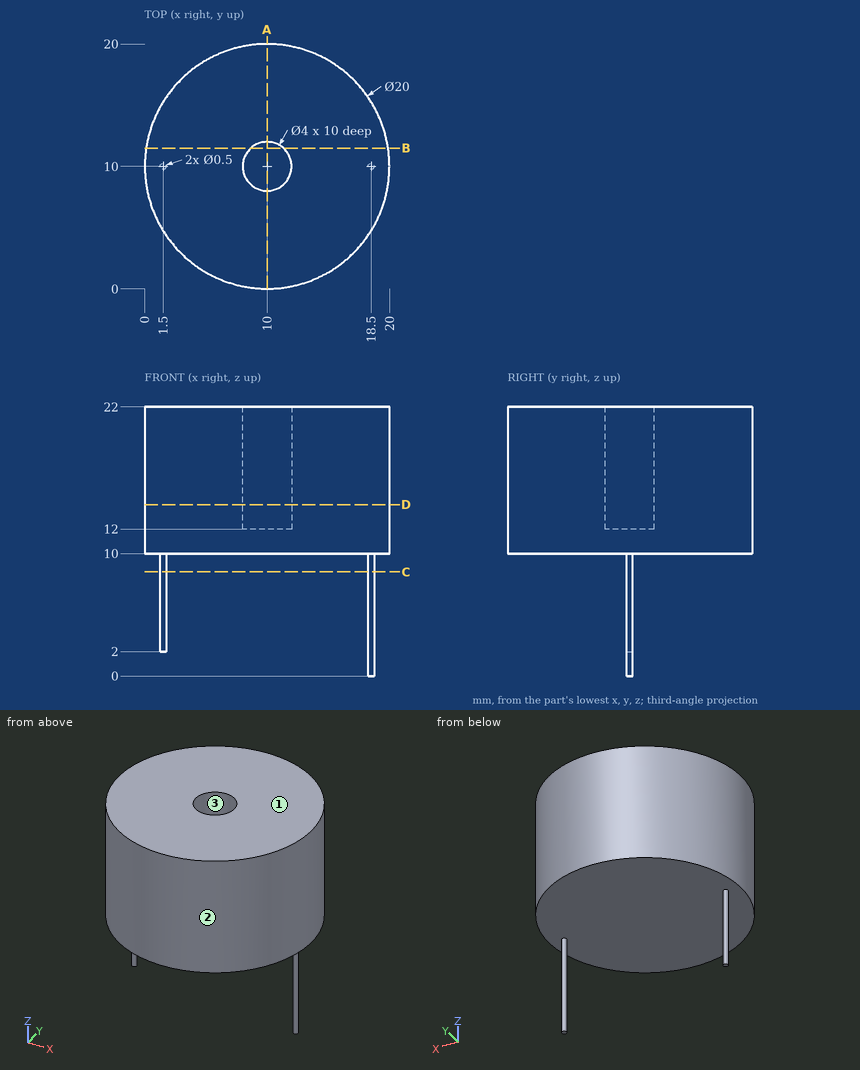
Print and shaded views of the part. All mm, measured from the part's lowest x, y and z. Give positions to 0.01 mm unless a question says otherwise; leave off trailing zeros. Write each loop counter-clockwise with the first axis right and the second up, starting at its lowest first coordinate (ties: lowest second). Pieces come first, ordered by that corner, then holes. Notation, with made-up numbers: (19.5, 84) -> (68.5, 84) arc R22 cw to (68.5, 121) -> close; hole circle Ø9 at (83.25, 42). An arc over 180 degrees is marked (long way). Use CSV: the item, a comma, the result in double quotes. Start each with the question number.
1) Cut at C-C on z = 8.5. List the corners of the cut face in (x, y), plus the area to 3 significant figures.
2) Cut at D-D on z = 14. List the corners of the cut face in (x, y), plus the area to 3 significant figures.
3) Pin check, flat tips, straight feed: P1, Ø12, axis at x = 7, z = 15.5, coming from the -Y side; P2, Ø12, axis at y = 17.5, z = 7.5, coming from the +X side; P3, Ø8, axis at x = 15.5, z = 8, coming from the -Y side; P4, Ø4, axis at y = 17, z = 16.5, coming from the +X side. Stop position of each tip, or through.
4) Drill centre lines: L1, parallel to Y at x = 10, z = 19; L2, parallel to Z at x = 3.75, y = 5.25; L3, parallel to Y at x = 18.5, z = 2. Where is each one in solid material? Low to high.
5) Two-plate mould, pull along Y, no slides. Class the marked faces 1, 2 and 3: released by +Y, released by -Y, zero draft, split by the parting line, or undercut.
6) Cut at A-A on x = 10. List the corners of the cut face in (y, z).
7) Cut at B-B on y = 11.5. List the corners of the cut face in (x, z).
Final values:
1,outline,"circle Ø0.5 at (1.5, 10); circle Ø0.5 at (18.5, 10)"
1,area,"0.393 mm2"
2,outline,"circle Ø20 at (10, 10); hole circle Ø4 at (10, 10)"
2,area,"302 mm2"
3,P1,"stops at y = 0"
3,P2,"stops at x = 19.79"
3,P3,"stops at y = 0.21"
3,P4,"stops at x = 18.66"
4,L1,"y = 0 to 8, 12 to 20"
4,L2,"z = 10 to 22"
4,L3,"y = 9.75 to 10.25"
5,face 1,"zero draft"
5,face 2,"split by the parting line"
5,face 3,"undercut"
6,outline,"(0, 10) -> (20, 10) -> (20, 22) -> (12, 22) -> (12, 12) -> (8, 12) -> (8, 22) -> (0, 22) -> close"
7,outline,"(0.11, 10) -> (19.89, 10) -> (19.89, 22) -> (11.32, 22) -> (11.32, 12) -> (8.68, 12) -> (8.68, 22) -> (0.11, 22) -> close"
